from build123d import *

# Parameters (mm, degrees)
BOSS_EXTRUDE1_DEPTH = 35
SKETCH2_R           = 9
BOSS_EXTRUDE2_DEPTH = 2
SKETCH3_R           = 4
CUT_EXTRUDE1_DEPTH  = 5
SKETCH4_W           = 5
SKETCH4_H           = 35
BOSS_EXTRUDE3_DEPTH = 20.5
SKETCH6_W           = 5
SKETCH6_H           = 25.5
BOSS_EXTRUDE4_DEPTH = 2.5
SKETCH7_W           = 5
SKETCH7_H           = 20
BOSS_EXTRUDE5_DEPTH = 7.5
SKETCH8_W           = 20
SKETCH8_H           = 5
BOSS_EXTRUDE6_DEPTH = 15
SKETCH10_W          = 10
SKETCH10_H          = 10
CUT_EXTRUDE2_DEPTH  = 5


with BuildPart() as part:
    # Sketch1 → Boss-Extrude1 (new body)
    with BuildSketch(Plane.XY):
        Polygon((-9.305574102, 4.73561153), (15.694425898, 4.73561153), (15.694425898, -0.26438847), (1.694425898, -0.26438847), (-4.305574102, -6.26438847), (-4.305574102, -13.26438847), (-9.305574102, -13.26438847), align=None)
    extrude(amount=BOSS_EXTRUDE1_DEPTH)

    # Sketch2 → Boss-Extrude2 (add)
    with BuildSketch(Plane(origin=(0, 4.73561153, 0), x_dir=(1, 0, 0), z_dir=(0, 1, 0))):
        with Locations((2.904425898, -17.63)):
            Circle(SKETCH2_R)
    extrude(amount=BOSS_EXTRUDE2_DEPTH)

    # Sketch3 → Cut-Extrude1 (cut)
    with BuildSketch(Plane(origin=(0, 6.73561153, 0), x_dir=(1, 0, 0), z_dir=(0, 1, 0))):
        with Locations((2.904425898, -17.63)):
            Circle(SKETCH3_R)
    extrude(amount=-CUT_EXTRUDE1_DEPTH, mode=Mode.SUBTRACT)

    # Sketch4 → Boss-Extrude3 (add)
    with BuildSketch(Plane.XZ.offset(0.26438847)):
        with Locations((13.194425898, 17.5)):
            Rectangle(SKETCH4_W, SKETCH4_H)
    extrude(amount=BOSS_EXTRUDE3_DEPTH)

    # Sketch6 → Boss-Extrude4 (add)
    with BuildSketch(Plane(origin=(15.694425898, 0, 0), x_dir=(0, 0, -1), z_dir=(1, 0, 0))):
        with Locations((-2.5, -8.01438847)):
            Rectangle(SKETCH6_W, SKETCH6_H)
    extrude(amount=BOSS_EXTRUDE4_DEPTH)

    # Sketch7 → Boss-Extrude5 (add)
    with BuildSketch(Plane.XZ.offset(13.26438847)):
        with Locations((-6.805574102, 25)):
            Rectangle(SKETCH7_W, SKETCH7_H)
    extrude(amount=BOSS_EXTRUDE5_DEPTH)

    # Sketch8 → Boss-Extrude6 (add)
    with BuildSketch(Plane(origin=(-4.305574102, 0, 0), x_dir=(0, 0, -1), z_dir=(1, 0, 0))):
        with Locations((-25, -18.26438847)):
            Rectangle(SKETCH8_W, SKETCH8_H)
    extrude(amount=BOSS_EXTRUDE6_DEPTH)

    # Sketch10 → Cut-Extrude2 (cut)
    with BuildSketch(Plane(origin=(15.694425898, 0, 0), x_dir=(0, 0, -1), z_dir=(1, 0, 0))):
        with Locations((-23, -5.26438847)):
            Rectangle(SKETCH10_W, SKETCH10_H)
    extrude(amount=-CUT_EXTRUDE2_DEPTH, mode=Mode.SUBTRACT)


solid = part.part
Verification items for the finished model (mm, model axes). A direction names the side the tool comes from. Coordinates: 2 decimals unless noted, no trailing zeros. Loops run counter-clockwise (first coordinate to the right, second up) from the corner with the lowest first, then second, coordinate; pieces in that order, holes last. Notation, with made-up numbers: (49, -24.5) -> (104, -24.5) arc R16 ccw to (104, -2.5) -> close; hole circle Ø10 at (-17, -23.5). An arc over 180 degrees is marked (long way). Write each question's results on one line, items separated by ' | '.
Item 1: Section check D-D, the plane y = -2.5. Enter the section's corners in (x, z), plus the area to 3 significant figures.
Found:
outline: (-9.31, 0) -> (-0.54, 0) -> (-0.54, 35) -> (-9.31, 35) -> close; (10.69, 0) -> (18.19, 0) -> (18.19, 5) -> (15.69, 5) -> (15.69, 18) -> (10.69, 18) -> close; (10.69, 28) -> (15.69, 28) -> (15.69, 35) -> (10.69, 35) -> close | area: 444 mm2
Item 2: Section check B-B, the plane y = -18. Enter the section's corners in (x, z).
Found:
outline: (-9.31, 15) -> (10.69, 15) -> (10.69, 0) -> (18.19, 0) -> (18.19, 5) -> (15.69, 5) -> (15.69, 35) -> (-9.31, 35) -> close
Item 3: Section check A-A, the plane x = 15. Enter the section's corners in (y, z).
Found:
outline: (-20.76, 0) -> (4.74, 0) -> (4.74, 35) -> (-20.76, 35) -> close; hole (-10.26, 18) -> (-0.26, 18) -> (-0.26, 28) -> (-10.26, 28) -> close
Item 4: Section check C-C, the plane z = 16. Enter the section's corners in (x, y).
Found:
outline: (-9.31, -20.76) -> (15.69, -20.76) -> (15.69, 4.74) -> (11.76, 4.74) -> (11.76, 6.74) -> (6.56, 6.74) -> (6.56, 1.74) -> (-0.75, 1.74) -> (-0.75, 6.74) -> (-5.95, 6.74) -> (-5.95, 4.74) -> (-9.31, 4.74) -> close; hole (-4.31, -15.76) -> (10.69, -15.76) -> (10.69, -0.26) -> (1.69, -0.26) -> (-4.31, -6.26) -> close
Item 5: Gauge pin test, flat ends, axial feed: pin 1 (5.5 mm diameter, centred on x = 12, z = 22.5, fed in from +Y); pin 2 (2.5 mm diameter, centred on x = 17, y = -14.5, fed in from +Z); pin 3 (1 mm diameter, centred on x = 13, z = 6, fed in from +Y); pin 4 (6 mm diameter, centred on x = 1, y = -5.5, fed in from -Z). Record the tip position at first contact, or that the pin passes through.
Found:
pin 1: stops at y = 6.74 | pin 2: stops at z = 5 | pin 3: stops at y = 4.74 | pin 4: passes through
Item 6: Tool access check on faces 1 (the face through (-3.73, 5.72, 11.55)), 2 (the face through (17, -8, 5)), 3 (the face through (13, -5, 18)), 4 (the face through (3, -15.764, 25)), 5 (the face through (1, -18, 15)). Record the directions out of +Z, -Z, +X, -X, +Y, -Y that give a thin tool (end or side, any length) a straight path to the whole face; none if there is none.
Found:
face 1: +Y | face 2: +Z, +X, +Y, -Y | face 3: +X | face 4: +Z, -Z | face 5: -Z, -X, -Y
Item 7: Mould release check, pull along Z, two halves, no side actions. Record for faces 6 (the face through (4, 0, 0)), 7 (the face through (-1.26, -3.22, 17.26)), 8 (the face through (3, 1.736, 18)): +Z half, -Z half, draft (parallel to the pull), parting line (faces both ways), or undercut.
Found:
face 6: -Z half | face 7: draft | face 8: undercut
Item 8: Material ranges on L1, parallel to X at y = 5.55, z = 17.63; L2, parallel to Y at x = 12, z = 25; L3, parallel to X at y = 3.8, z = 17.63, recorded low to high.
Found:
L1: x = -6.1 to -1.1, 6.9 to 11.9 | L2: y = -20.76 to -10.26, -0.26 to 4.74 | L3: x = -9.31 to -1.1, 6.9 to 15.69
